Geometry: final body of the model. Coordinates: model frame, mm. Give positions to 0.01 mm unless a question says otherwise; leave off trailing zeros. Write each loop counter-clockwise with the first axis right and the second up, starting at its lowest first coordinate (ties: lowest second). Pieces come first, ordered by that corner, then holes.
from build123d import *

# Parameters (mm, degrees)
F0_W     = 21.434508
F0_H     = 0.762
F1_DEPTH = 40.64
F0_W_2   = 11.613984
F2_DEPTH = 48.26


with BuildPart() as f1:
    # F0 (on Top) → F1 (new body)
    with BuildSketch(Plane.XY):
        with Locations((16.524246, 0)):
            Rectangle(F0_W, F0_H)
        with Locations((-16.524246, 0)):
            Rectangle(F0_W, F0_H)
    extrude(amount=F1_DEPTH)

    # F0 (on Top) → F2 (join)
    with BuildSketch(Plane.XY):
        Rectangle(F0_W_2, F0_H)
    extrude(amount=F2_DEPTH)


solid = f1.part
Q1. Section B-B on x = 9. Output: boundary loops of the cut face in (y, z), plus the area to 3 significant figures.
Filled sheet:
outline: (-0.38, 0) - (0.38, 0) - (0.38, 40.64) - (-0.38, 40.64) - close
area: 31.0 mm2
Q2. Section A-A on y = 0.2. Output: boundary loops of the cut face in (x, z), plus the area to 3 significant figures.
Filled sheet:
outline: (-27.24, 0) - (27.24, 0) - (27.24, 40.64) - (5.81, 40.64) - (5.81, 48.26) - (-5.81, 48.26) - (-5.81, 40.64) - (-27.24, 40.64) - close
area: 2,300 mm2
Q3. Ray query, line 1 along Z through (x, y) = (20.5, 0); line 2 along X through (y, z) = (-0.2, 45.5). Return the intervals inside material, ascending.
Filled sheet:
line 1: z = 0 to 40.64
line 2: x = -5.81 to 5.81
Q4. Section C-C on z = 45.5. Output: boundary loops of the cut face in (x, y).
Filled sheet:
outline: (-5.81, -0.38) - (5.81, -0.38) - (5.81, 0.38) - (-5.81, 0.38) - close
